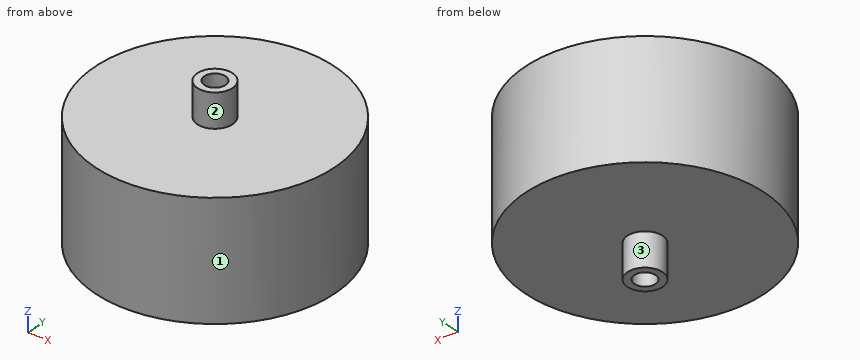
Autodesk Inventor part; units mm, degrees
ref_plane "YZ Plane" through (0, 0, 0) normal (1, 0, 0) x (0, 1, 0)
ref_plane "XZ Plane" through (0, 0, 0) normal (0, 1, 0) x (-1, 0, 0)
ref_plane "XY Plane" through (0, 0, 0) normal (0, 0, 1) x (1, 0, 0)
sketch "スケッチ1" plane through (0, 0, 0) normal (0, 0, 1) x (1, 0, 0)
  circle A0 centre (0, 0) radius 68
  dimension "d0" = 136
extrude "押し出し1" add sketch "スケッチ1" along normal mid plane 66
sketch "スケッチ2" plane through (0, 0, 0) normal (0, 0, 1) x (1, 0, 0)
  circle A0 centre (0, 0) radius 10
  dimension "d3" = 20
extrude "押し出し2" add sketch "スケッチ2" along normal mid plane 104
sketch "スケッチ3" plane through (0, 0, 52) normal (0, 0, 1) x (1, 0, 0)
  point P0 (0, 0)
  point P1 (0, 0)
hole "穴1" at (0, 0, 52) direction (0, 0, -1) diameter 12 end through all
properties part number "前輪ハブ"
Could you check a few things on this model? Use its own coordinates, in mm. Face numbers are marked on the shaded views. A direction names the side the tool comes from. Give positions to 0.01 mm unless a question says otherwise; leave off trailing zeros. Order: outer loops, then holes, each group sorted by start corner. A loop starts at its lowest first (then second) coordinate and runs counter-clockwise, first axis right, second up. Notation, with made-up numbers: (-10, 18) -> (10, 18) arc R13 cw to (10, 29) -> close; hole circle Ø5 at (-18, 51.25). An arc over 180 degrees is marked (long way). Answer in a Markdown table with one row per item. Add a question column.
Item 1: I'm going to push flat-ended pins straight in: P1, Ø19, axis at x = 0, y = 0, coming from the +Z side; P2, Ø8, axis at x = -39.5, z = 2, coming from the -Y side; P3, Ø5, axis at x = 43.5, z = -21, coming from the -Y side; P4, Ø1.5, axis at x = -13.5, y = -44, coming from the +Z side. Where does each tip first touch, or does it pass through?
Item 2: Imagine slicing it at D-D (x = -52). List the corners of the cut face in (y, z) for me.
Item 3: Imagine slicing it at C-C (z = -31). List the corners of the cut face in (x, y) for me.
Item 4: For the marked faces 1, 2 and 3, which set-ups out of +Z, -Z, +X, -X, +Y, -Y let a thin tool reach every point of the face, with its end or its side?
Item 5: Please list where these lines run through material, in increasing order: probe 1 along Y at (x, z) = (0, -14.5); probe 2 along Z at (x, y) = (-22, 43); probe 3 along Y at (x, z) = (9, 15).
Item 6: Imagine slicing it at A-A (y = 0). List the corners of the cut face in (x, z) for me, and give its area (3 significant figures).
Result:
| question | item | result |
|---|---|---|
| 1 | P1 | z = 52 |
| 1 | P2 | y = -58 |
| 1 | P3 | y = -54.25 |
| 1 | P4 | z = 33 |
| 2 | outline | (-43.82, -33) -> (43.82, -33) -> (43.82, 33) -> (-43.82, 33) -> close |
| 3 | outline | circle Ø136 at (0, 0); hole circle Ø12 at (0, 0) |
| 4 | face 1 | +Z, -Z |
| 4 | face 2 | +Z |
| 4 | face 3 | -Z |
| 5 | probe 1 | -68 to -6, 6 to 68 |
| 5 | probe 2 | -33 to 33 |
| 5 | probe 3 | -67.4 to 67.4 |
| 6 | outline | (-68, -33) -> (-10, -33) -> (-10, -52) -> (-6, -52) -> (-6, 52) -> (-10, 52) -> (-10, 33) -> (-68, 33) -> close; (6, -52) -> (10, -52) -> (10, -33) -> (68, -33) -> (68, 33) -> (10, 33) -> (10, 52) -> (6, 52) -> close |
| 6 | area | 8,490 mm2 |
